Design review of the part built by this model. Coordinates are the model's own, in mm. Face numbers are marked on the shaded views. A direction names the side the tool comes from. Give positions to 0.01 mm unless a question says otherwise; leave off trailing zeros. Order: outer loops, then holes, each group sorted by start corner. A loop starts at its lowest first (then second) coordinate and runs counter-clockwise, first axis right, second up. Notation, with made-up numbers: (26, 18.5) -> (74, 18.5) arc R12 ccw to (74, 22.5) -> close; hole circle Ø5 at (44.25, 28). An arc over 180 degrees is marked (long way). One line per item, written item: value. Start each with the question number.
1) Consider section C-C (y = 10.75). State the section outline as (x, z) points, plus the area to 3 significant figures.
2) The part is to be moulded in two halves that separate along Y. For the marked faces 1, 2, 3 and 4, say which applies: released by +Y, released by -Y, zero draft, split by the parting line, or undercut.
3) Wall thickness on line 1 along Z through (x, y) = (0, 12.75); line 2 along Z through (x, y) = (0, 4.75): over which ranges is each line inside the solid? List them lowest first. Write a range as from..to.
4) For pin 1 (1 mm diameter, centred on y = 10, z = -3, fed in from +X); pin 2 (5 mm diameter, centred on x = -7, z = -12, fed in from +Y); pin 3 (6 mm diameter, centred on x = -6.5, y = 11, fed in from +Z), all flat-tipped, find the tip position at first contact; note any pin that passes through.
5) Consider section A-A (x = 0). State the section outline as (y, z) points.
6) Tool access review of the marked faces 5, 6 and 7: name each direction out of +Z, -Z, +X, -X, +Y, -Y from which nothing blocks a thin tool from reaching the whole face with its end or side.
7) Consider section B-B (z = 0). State the section outline as (x, y) points, plus the area to 3 significant figures.
from build123d import *

# Parameters (mm, degrees)
CYLINDER_R     = 1.5
CYLINDER_DEPTH = 22


with BuildPart() as cylinder:
    # Cylinder → Cylinder (new body)
    with BuildSketch(Plane(origin=(0, 18, -11), x_dir=(1, 0, 0), z_dir=(0, 0, 1))):
        Circle(CYLINDER_R)
    extrude(amount=CYLINDER_DEPTH)


with BuildPart() as cut:
    # Sketch → Revolve (revolve)
    with BuildSketch(Plane.XY):
        Polygon((4.05, 0), (4.05, 18), (10.05, 18), (10.05, 8.389587), (18, 8.389587), (9.909247, 5.444793), (9.909247, 2.944793), (18, 0), align=None)
    revolve(axis=Axis((0, 0, 0), (0, 1, 0)))

    # Cut: cut Cylinder
    add(cylinder.part, mode=Mode.SUBTRACT)


solid = cut.part
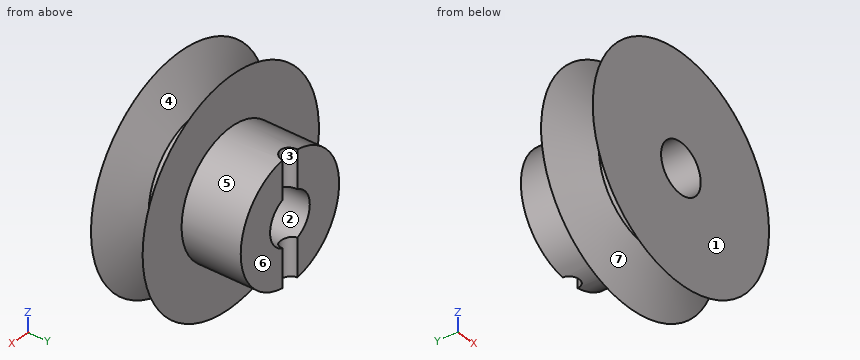
Checked values:
1. outline: circle Ø20.1 at (0, 0); hole circle Ø8.1 at (0, 0)
1. area: 266 mm^2
2. face 1: released by -Y
2. face 2: zero draft
2. face 3: released by +Y
2. face 4: undercut
3. line 1: z = -10.05..-4.05, 4.05..10.05
3. line 2: z = -9.91..-4.05, 4.05..9.91
4. pin 1: stops at x = 9.73
4. pin 2: stops at y = 8.39
4. pin 3: stops at z = 17.29
5. outline: (0, -18) -> (2.94, -9.91) -> (5.44, -9.91) -> (8.39, -18) -> (8.39, -10.05) -> (16.5, -10.05) -> (16.5, -4.05) -> (0, -4.05) -> close; (0, 4.05) -> (16.5, 4.05) -> (16.5, 10.05) -> (8.39, 10.05) -> (8.39, 18) -> (5.44, 9.91) -> (2.94, 9.91) -> (0, 18) -> close
6. face 5: +Y
6. face 6: +Z, -Z, +X, -X, +Y
6. face 7: none
7. outline: (-18, 0) -> (-4.05, 0) -> (-4.05, 18) -> (-10.05, 18) -> (-10.05, 8.39) -> (-18, 8.39) -> (-9.91, 5.44) -> (-9.91, 2.94) -> close; (4.05, 0) -> (18, 0) -> (9.91, 2.94) -> (9.91, 5.44) -> (18, 8.39) -> (10.05, 8.39) -> (10.05, 18) -> (4.05, 18) -> close
7. area: 261 mm^2
